CAD build for the part. Positions are in the model's coordinates, mm. A direction names the side the tool comes from. Round coordinates to 2 decimals unless told otherwise and drop trailing zeros. Loops run counter-clockwise (first coordinate to the right, second up) from the corner with the lowest first, then second, coordinate; pieces in that order, holes last.
from build123d import *

# Parameters (mm, degrees)
CROQUIS1_W              = 100
CROQUIS1_H              = 70
SALIENTE_EXTRUIR1_DEPTH = 5
CROQUIS3_R              = 2
CORTAR_EXTRUIR2_DEPTH   = 6
CROQUIS6_R              = 2
CORTAR_EXTRUIR3_DEPTH   = 6
CROQUIS7_W              = 25
CROQUIS7_H              = 54
CORTAR_EXTRUIR4_DEPTH   = 6
CORTAR_EXTRUIR5_DEPTH   = 6
CHAFL_N1_SIZE           = 1


with BuildPart() as part:
    # Croquis1 → Saliente-Extruir1 (new body)
    with BuildSketch(Plane(origin=(0, 0, 0), x_dir=(1, 0, 0), z_dir=(0, 1, 0))):
        Rectangle(CROQUIS1_W, CROQUIS1_H)
    extrude(amount=SALIENTE_EXTRUIR1_DEPTH)

    # Croquis3 → Cortar-Extruir2 (cut, through all)
    with BuildSketch(Plane(origin=(0, 5, 0), x_dir=(1, 0, 0), z_dir=(0, 1, 0))):
        with Locations((-44, 29)):
            Circle(CROQUIS3_R)
        with Locations((44, 29)):
            Circle(CROQUIS3_R)
        with Locations((44, -29)):
            Circle(CROQUIS3_R)
        with Locations((-44, -29)):
            Circle(CROQUIS3_R)
    extrude(amount=-CORTAR_EXTRUIR2_DEPTH, mode=Mode.SUBTRACT)

    # Croquis6 → Cortar-Extruir3 (cut, through all)
    with BuildSketch(Plane(origin=(0, 5, 0), x_dir=(1, 0, 0), z_dir=(0, 1, 0))):
        with Locations((-10, 0)):
            Circle(CROQUIS6_R)
        with Locations((10, 0)):
            Circle(CROQUIS6_R)
    extrude(amount=-CORTAR_EXTRUIR3_DEPTH, mode=Mode.SUBTRACT)

    # Croquis7 → Cortar-Extruir4 (cut, through all)
    with BuildSketch(Plane.XZ):
        with Locations((-27.5, 0)):
            Rectangle(CROQUIS7_W, CROQUIS7_H)
        with Locations((27.5, 0)):
            Rectangle(CROQUIS7_W, CROQUIS7_H)
    extrude(amount=-CORTAR_EXTRUIR4_DEPTH, mode=Mode.SUBTRACT)

    # Croquis8 → Cortar-Extruir5 (cut, through all)
    with BuildSketch(Plane(origin=(0, 5, 0), x_dir=(1, 0, 0), z_dir=(0, 1, 0))):
        Polygon((-10, 35), (0, 20), (10, 35), align=None)
    cortar_extruir5 = extrude(amount=-CORTAR_EXTRUIR5_DEPTH, mode=Mode.SUBTRACT)

    # Simetría1: Cortar-Extruir5 across plane
    add(cortar_extruir5.mirror(Plane.XY), mode=Mode.SUBTRACT)

    # Chaflán1
    chafl_n1_edges = [part.edges().sort_by_distance(p)[0] for p in [
        (-46, 5, 29),
        (42, 5, 29),
        (42, 5, -29),
        (-46, 5, -29),
        (-12, 5, 0),
        (8, 5, 0),
        (-15, 5, 0),
        (-27.5, 5, -27),
        (-40, 5, 0),
        (-27.5, 5, 27),
        (40, 5, 0),
        (27.5, 5, -27),
        (15, 5, 0),
        (27.5, 5, 27),
    ]]
    chamfer(chafl_n1_edges, length=CHAFL_N1_SIZE)


solid = part.part
Item 1: Mould opens along Z. For faces 1 (the flat face through (15, 2, 0)), 2 (the flat face through (-50, 2, 0)), 3 (the cylindrical face through (44, 2, 31)), 4 (the flat face through (-5.07, 2.535, -27.605)) say: released by +Z, released by -Z, zero draft, split by the parting line, or undercut.
Verdict:
face 1: undercut
face 2: zero draft
face 3: undercut
face 4: released by -Z
Item 2: Cut at D-D (x = 22). List the corners of the cut face in (y, z).
Verdict:
outline: (0, -35) - (5, -35) - (5, -28) - (4, -27) - (0, -27) - close; (0, 27) - (4, 27) - (5, 28) - (5, 35) - (0, 35) - close
Item 3: Cut at B-B (y = 3.05). State how many separate pieces and enclosed holes the cut face has, plus the area to 3 significant figures.
Verdict:
separate pieces: 1
enclosed holes: 8
area: 3,920 mm2
Item 4: Wall check: L1, parallel to X at y = 1.1, z = -5; L2, parallel to X at y = 2.05, z = 0; L3, parallel to Z at x = -44, y = 2.4. Give the ranges that are in metal, low to high.
Verdict:
L1: x = -50 to -40, -15 to 15, 40 to 50
L2: x = -50 to -40, -15 to -12, -8 to 8, 12 to 15, 40 to 50
L3: z = -35 to -31, -27 to 27, 31 to 35
Item 5: Cut at A-A (x = 44). List the corners of the cut face in (y, z).
Verdict:
outline: (0, -35) - (5, -35) - (5, -32) - (4, -31) - (0, -31) - close; (0, -27) - (4, -27) - (5, -26) - (5, 26) - (4, 27) - (0, 27) - close; (0, 31) - (4, 31) - (5, 32) - (5, 35) - (0, 35) - close
Item 6: Cut at C-C (z = 7). List the corners of the cut face in (x, y).
Verdict:
outline: (-50, 0) - (-40, 0) - (-40, 4) - (-41, 5) - (-50, 5) - close; (-15, 0) - (15, 0) - (15, 4) - (14, 5) - (-14, 5) - (-15, 4) - close; (40, 0) - (50, 0) - (50, 5) - (41, 5) - (40, 4) - close
Item 7: 3-axis set-ups, long thin cutter, end or side, ignore diameter. For faces 5 (the flat face through (4.93, 2.535, 27.395)), 6 (the flat face through (4.93, 2.535, -27.395)), 7 (the flat face through (-1, 0, 0)), 8 (the flat face through (30, 2, 35)), 9 (the flat face through (-15, 2, 0)): which of +Z, -Z, +X, -X, +Y, -Y reach the whole face in a straight line?
Verdict:
face 5: +Z, +Y, -Y
face 6: -Z, +Y, -Y
face 7: +Z, -Z, +X, -X, -Y
face 8: +Z, +X, -X, +Y, -Y
face 9: +Y, -Y
Item 8: Flat gauge pins, fed straight in: P1, Ø4.5, axis at x = 44, z = 29, coming from the +Y side; P2, Ø3.5, axis at x = 10, z = 0, coming from the +Y side. Where does each tip first touch, or does it go through?
Verdict:
P1: stops at y = 4.25
P2: passes through
